Can you work these out from the drawing? Everything is in mm from the part's minimum corner. A direction names the side the tool comes from. Round coordinates to 2 decimals unless told otherwise and drop trailing zeros. Write each loop counter-clockwise with the first axis right and the second up, starting at its lowest first coordinate (ties: lowest second). Pieces come first, ordered by that corner, then holes. Notation, with made-up numbers: M 24.25,-30 L 32.25,-30 A11 ccw 32.25,-25 Z; hole C -23,-19 d1. An arc over 180 degrees is marked long. Answer in a Markdown table with one row per item. Add a question column.
(1) Suppose I cut it at B-B, the plane y = 29. Write out the boundary of the cut face in (x, z).
(2) Suppose I cut it at A-A, the plane z = 9. Write out the boundary of the cut face in (x, y), then the cut area to 3 significant figures.
(3) For the marked faces 4, 5 and 6, which set-ups out of +Z, -Z, +X, -X, +Y, -Y let a thin tool reach every point of the face, with its end or its side?
(4) I'm going to push flat-ended pins straight in: pin 1 (12.5 mm diameter, centred on y = 40, z = 57, fed in from +X); pin 2 (8 mm diameter, centred on y = 41, z = 6.5, fed in from -X); pin 3 (12.5 mm diameter, centred on x = 83, y = 46.5, fed in from +Z); pin 4 (7.5 mm diameter, centred on y = 46, z = 53, fed in from -X). Where does each tip first touch, or does it pass through?
(5) Suppose I cut it at D-D, the plane z = 46.5. Write out the boundary of the cut face in (x, y).
(6) Suppose I cut it at C-C, the plane x = 21. Write out the boundary of the cut face in (y, z).
(7) If we mould it in two halves opening along X, with no side actions, what happens to the marked faces 1, 2 and 3? For each: released by +X, released by -X, zero draft, split by the parting line, or undercut.
(8) If I drill on probe 1 along Z at (x, y) = (17, 29.5); probe 2 along X at (y, z) = (54.5, 3.5); probe 3 along X at (y, z) = (60, 42.5), over which ranges is the centre line in solid material (lowest first)?
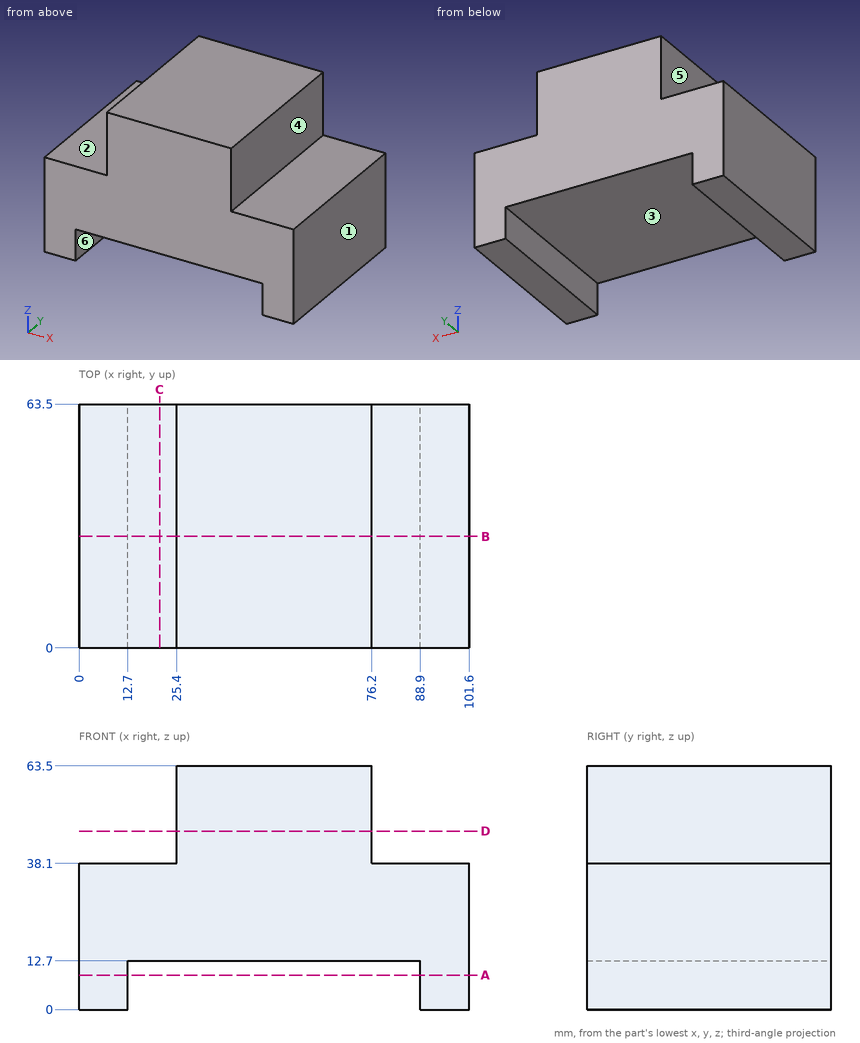
Calculated:
| question | item | result |
|---|---|---|
| 1 | outline | M 0,0 L 12.7,0 L 12.7,12.7 L 88.9,12.7 L 88.9,0 L 101.6,0 L 101.6,38.1 L 76.2,38.1 L 76.2,63.5 L 25.4,63.5 L 25.4,38.1 L 0,38.1 Z |
| 2 | outline | M 0,0 L 12.7,0 L 12.7,63.5 L 0,63.5 Z; M 88.9,0 L 101.6,0 L 101.6,63.5 L 88.9,63.5 Z |
| 2 | area | 1,610 mm² |
| 3 | face 4 | +Z, +X, +Y, -Y |
| 3 | face 5 | +Z, -X, +Y, -Y |
| 3 | face 6 | -Z, +Y, -Y |
| 4 | pin 1 | x = 76.2 |
| 4 | pin 2 | x = 0 |
| 4 | pin 3 | z = 38.1 |
| 4 | pin 4 | x = 25.4 |
| 5 | outline | M 25.4,0 L 76.2,0 L 76.2,63.5 L 25.4,63.5 Z |
| 6 | outline | M 0,12.7 L 63.5,12.7 L 63.5,38.1 L 0,38.1 Z |
| 7 | face 1 | released by +X |
| 7 | face 2 | zero draft |
| 7 | face 3 | undercut |
| 8 | probe 1 | 12.7 to 38.1 |
| 8 | probe 2 | 0 to 12.7, 88.9 to 101.6 |
| 8 | probe 3 | 25.4 to 76.2 |
